Could you check a few things on this drawing? It's one solid part, dimensions in mm from its lowest x, y, z. A direction names the side the tool comes from. Round coordinates to 2 decimals unless told otherwise and drop trailing zeros. Write each loop counter-clockwise with the first axis right and the second up, starting at its lowest first coordinate (ties: lowest second). Pieces come first, ordered by that corner, then holes. Notation, with made-up numbers: M 35.25,-37.75 L 53.25,-37.75 A30 cw 53.25,-12.75 Z; hole C 7.25,-27 d4. An arc over 180 degrees is marked long. One line per item, written item: value. Start each with the question number.
(1) Which directions (+Z, -Z, +X, -X, +Y, -Y) give clear straight access to the entire face, cutting with the end or side of a thin tool? Please do the marked faces 1, 2 and 3.
(2) I want a section at D-D on z = 34.5. Please give me the cut outline in (x, y).
(3) I want a section at B-B on y = 14. Please give me the cut outline in (x, z) (1 decimal).
(4) I want a section at C-C on x = 95. Please give me the cut outline in (y, z).
(5) If I drill on L1, parallel to Z at x = 51, y = 51.5; L2, parallel to Y at x = 6, z = 11 (1 decimal); L3, parallel to Z at x = 38, y = 5, over which ranges is the centre line in solid material (lowest first)?
(6) Thinking about a two-plate mould opening in Y: for the marked faces 4, 5 and 6, which applies, released by +Y, released by -Y, zero draft, split by the parting line, or undercut?
(7) I'm going to push flat-ended pins straight in: pin 1 Ø7.5 at (x, y) = (9.3, 10.18) entering from +Z; pin 2 Ø4 at (y, z) = (49.5, 13) entering from -X; pin 3 Ø4 at (y, z) = (39.5, 43) entering from -X. Where does each tip first touch, or does it pass through?
(8) I want a section at A-A on y = 38.1. Please give me the cut outline in (x, z).
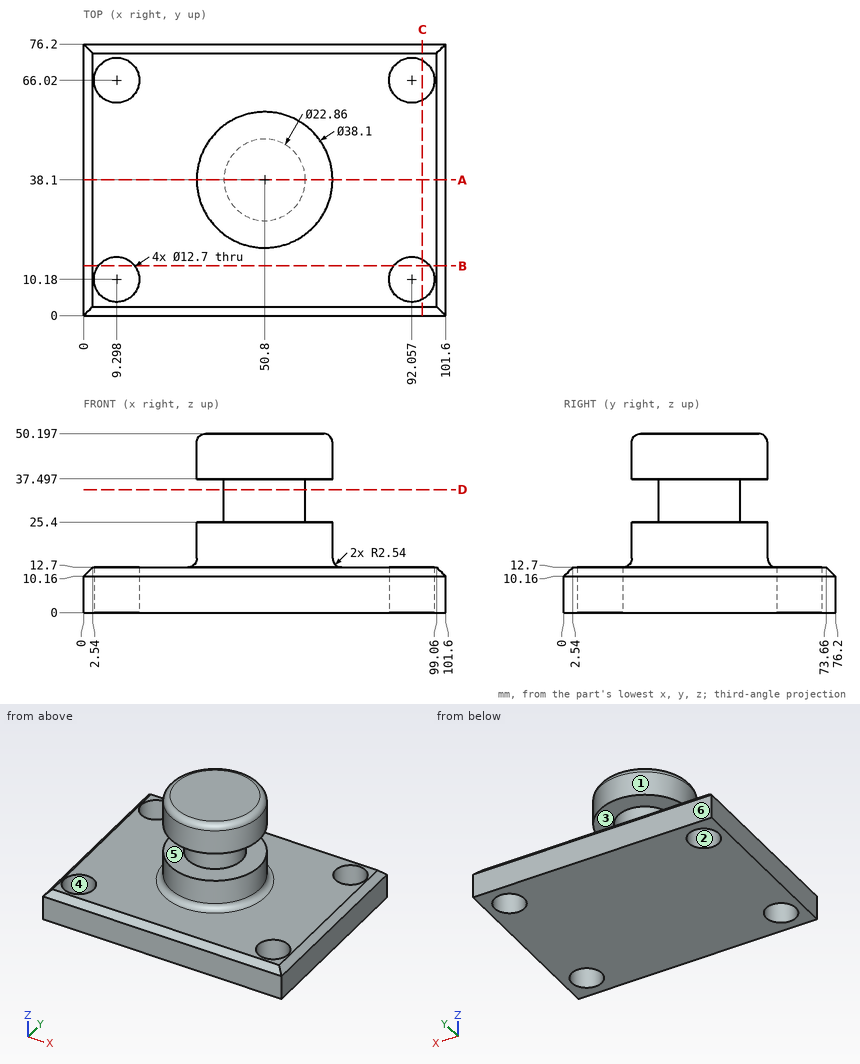
Found:
1. face 1: +Z
1. face 2: +Z, -Z
1. face 3: none
2. outline: C 50.8,38.1 d22.86
3. outline: M 0,0 L 4.2,0 L 4.2,12.7 L 2.5,12.7 L 0,10.2 Z; M 14.4,0 L 87,0 L 87,12.7 L 14.4,12.7 Z; M 97.1,0 L 101.6,0 L 101.6,10.2 L 99.1,12.7 L 97.1,12.7 Z
4. outline: M 0,0 L 4.55,0 L 4.55,12.7 L 2.54,12.7 L 0,10.16 Z; M 15.81,0 L 60.39,0 L 60.39,12.7 L 15.81,12.7 Z; M 71.65,0 L 76.2,0 L 76.2,10.16 L 73.66,12.7 L 71.65,12.7 Z
5. L1: z = 0 to 25.4, 37.5 to 50.2
5. L2: y = 0.8 to 4.8, 15.6 to 60.6, 71.4 to 75.4
5. L3: z = 0 to 12.7
6. face 4: undercut
6. face 5: zero draft
6. face 6: released by +Y
7. pin 1: passes through
7. pin 2: stops at x = 0.84
7. pin 3: stops at x = 31.75
8. outline: M 0,0 L 101.6,0 L 101.6,10.16 L 99.06,12.7 L 72.39,12.7 A2.54 cw 69.85,15.24 L 69.85,25.4 L 62.23,25.4 L 62.23,37.5 L 69.85,37.5 L 69.85,47.66 A2.54 ccw 67.31,50.2 L 34.29,50.2 A2.54 ccw 31.75,47.66 L 31.75,37.5 L 39.37,37.5 L 39.37,25.4 L 31.75,25.4 L 31.75,15.24 A2.54 cw 29.21,12.7 L 2.54,12.7 L 0,10.16 Z
